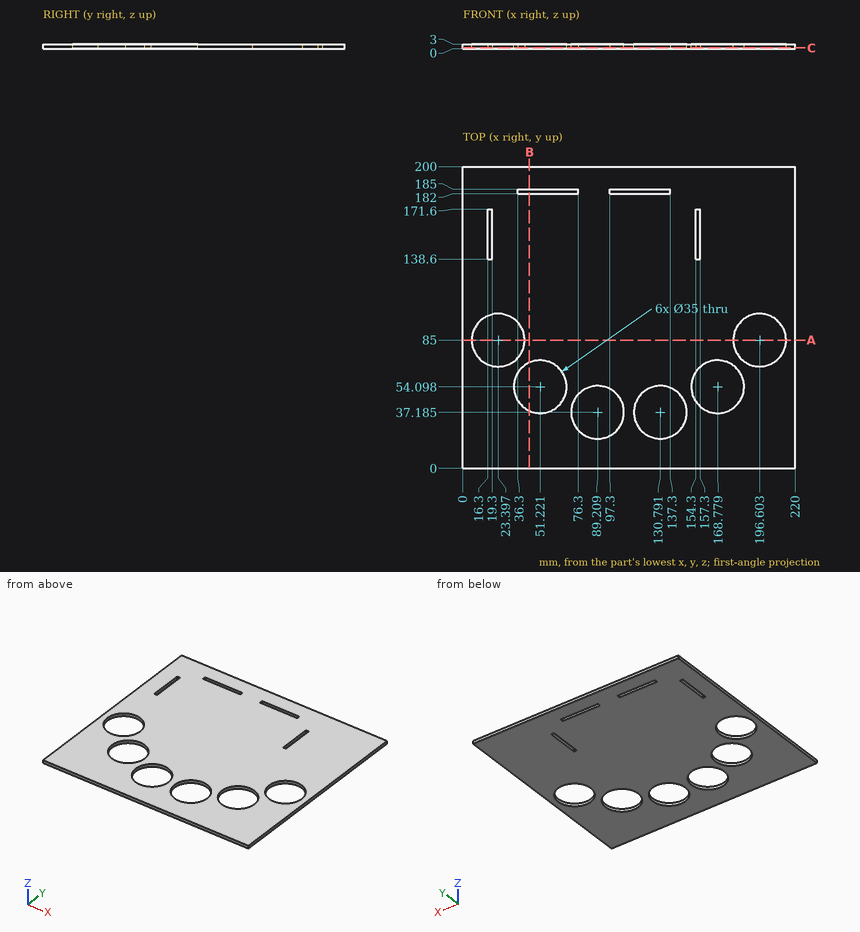
Design review of the part shown in the three views and the two pictorial views. Dimensions are in mm from the part's minimum x, y and z. Round coordinates to 2 decimals unless told otherwise and drop trailing zeros. Loops run counter-clockwise (first coordinate to the right, second up) from the corner with the lowest first, then second, coordinate; pieces in that order, holes last. Notation, with made-up numbers: (-35, -26) -> (-23, -26) arc R25 ccw to (-23, 8) -> close; hole circle Ø11 at (58, 81.25). An arc over 180 degrees is marked (long way). Return JSON: item names as keys, results as strings.
(1) Add section C-C on z = 0.5. State how many separate pieces and enclosed holes the cut face has, plus the area to 3 significant figures.
Solved:
{"separate pieces": "1", "enclosed holes": "10", "area": "37,800 mm2"}
(2) Add section B-B on x = 44. Write out the cut boundary in (y, z).
Solved:
{"outline": "(0, 0) -> (38.16, 0) -> (38.16, 3) -> (0, 3) -> close; (70.04, 0) -> (182, 0) -> (182, 3) -> (70.04, 3) -> close; (185, 0) -> (200, 0) -> (200, 3) -> (185, 3) -> close"}
(3) Add section A-A on y = 85. Write out the cut boundary in (x, z), plus the area to 3 significant figures.
Solved:
{"outline": "(0, 0) -> (5.9, 0) -> (5.9, 3) -> (0, 3) -> close; (40.9, 0) -> (179.1, 0) -> (179.1, 3) -> (40.9, 3) -> close; (214.1, 0) -> (220, 0) -> (220, 3) -> (214.1, 3) -> close", "area": "450 mm2"}
(4) For line 1 (X direction, y = 141.5, z = 0.6); line 2 (X direction, y = 184.5, z = 2.55); line 3 (Y direction, x = 22, z = 0.1) (1 decimal), list the stretches that pass through material, from the lowest coordinate up.
Solved:
{"line 1": "0 to 16.3, 19.3 to 154.3, 157.3 to 220", "line 2": "0 to 36.3, 76.3 to 97.3, 137.3 to 220", "line 3": "0 to 67.6, 102.4 to 200"}
